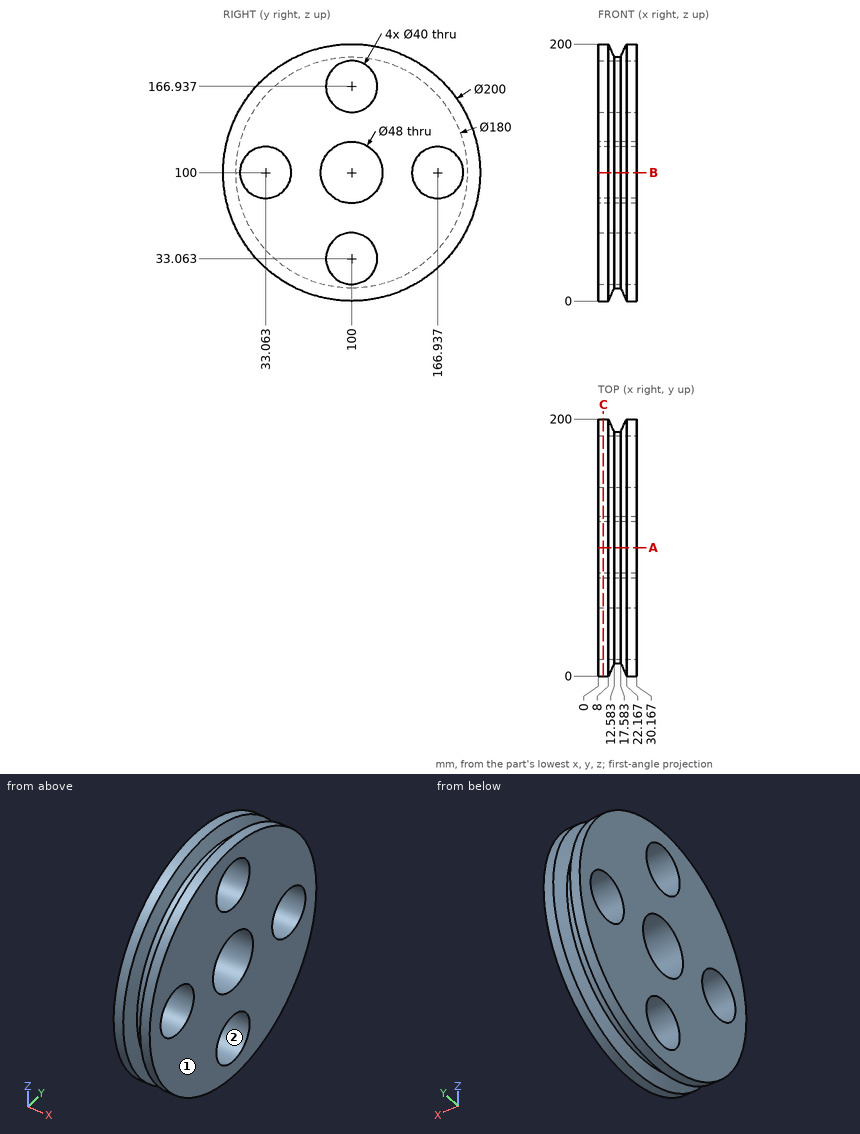
Input: dimensioned drawing with shaded views. Units: mm. Origin: part minimum x, y, z. Coordinates: 2 decimals unless noted, no trailing zeros. Loops run counter-clockwise (first coordinate to the right, second up) from the corner with the lowest first, then second, coordinate; pieces in that order, holes last. Notation, with made-up numbers: (14, 82.5) -> (70, 82.5) arc R31 cw to (70, 111.5) -> close; hole circle Ø5 at (0.25, 17.25). An arc over 180 degrees is marked (long way). Use a Markdown table: item, result. Add a question column.
(1) Section query A-A, the plane y = 100. Return loops of the section in (x, z).
(2) Line query: line 1 along Y through (x, z) = (15.5, 100); line 2 along Y through (x, z) = (24.5, 84) (1 decimal); line 3 along Z through (x, y) = (1, 107) (1 decimal). Output: solid intervals per line, ascending.
(3) Pin query (flat end, axial travel): pin 1 Ø24 at (y, z) = (100, 166.94) entering from -X; pin 2 Ø12 at (x, y) = (20, 131) entering from +Z; pin 3 Ø1.5 at (x, y) = (25, 27.5) entering from +Z (1 decimal). Return the tip coordinate at first contact, or that it passes through.
(4) Mould query, pull axis Y, two halves, no side actions, for the marked faces 1 and 2. Classes: pulls with the +Y half, pulls with the -Y half, needs draft (parallel to the pull), parting line crosses it, or undercut.
(5) Section query C-C, the plane x = 4. Return loops of the section in (y, z).
Answer:
| question | item | result |
|---|---|---|
| 1 | outline | (0, 0) -> (8, 0) -> (12.58, 10) -> (17.58, 10) -> (22.17, 0) -> (30.17, 0) -> (30.17, 13.06) -> (0, 13.06) -> close; (0, 53.06) -> (30.17, 53.06) -> (30.17, 76) -> (0, 76) -> close; (0, 124) -> (30.17, 124) -> (30.17, 146.94) -> (0, 146.94) -> close; (0, 186.94) -> (30.17, 186.94) -> (30.17, 200) -> (22.17, 200) -> (17.58, 190) -> (12.58, 190) -> (8, 200) -> (0, 200) -> close |
| 2 | line 1 | y = 10 to 13.06, 53.06 to 76, 124 to 146.94, 186.94 to 190 |
| 2 | line 2 | y = 1.3 to 21.1, 45.1 to 82.1, 117.9 to 154.9, 178.9 to 198.7 |
| 2 | line 3 | z = 0.2 to 14.3, 51.8 to 77, 123 to 148.2, 185.7 to 199.8 |
| 3 | pin 1 | passes through |
| 3 | pin 2 | stops at z = 196.72 |
| 3 | pin 3 | stops at z = 169.7 |
| 4 | face 1 | needs draft |
| 4 | face 2 | undercut |
| 5 | outline | circle Ø200 at (100, 100); hole circle Ø40 at (33.06, 100); hole circle Ø48 at (100, 100); hole circle Ø40 at (100, 33.06); hole circle Ø40 at (100, 166.94); hole circle Ø40 at (166.94, 100) |
